```python
from build123d import *

# Parameters (mm, degrees)
BOSS_EXTRUDE1_DEPTH = 2
BOSS_EXTRUDE2_DEPTH = 22.5
SKETCH1_6_R         = 2.2
SKETCH1_6_R_2       = 1.3
BOSS_EXTRUDE3_DEPTH = 25
CUT_EXTRUDE1_DEPTH  = 25
SKETCH3_R           = 1.5
CUT_EXTRUDE2_DEPTH  = 25


with BuildPart() as part:
    # Sketch1 → Boss-Extrude1 (new body)
    with BuildSketch(Plane.XY):
        Polygon((-5, -5), (93, -5), (93, 0), (93, 56), (93, 61), (-5, 61), align=None)
    extrude(amount=BOSS_EXTRUDE1_DEPTH)

    # Sketch1_5 → Boss-Extrude2 (add)
    with BuildSketch(Plane.XY):
        with BuildLine():
            Line((-5, 63), (93, 63))
            ThreePointArc((93, 63), (94.414213562, 62.414213562), (95, 61))
            Line((95, 61), (95, 56))
            Line((95, 56), (95, 0))
            Line((95, 0), (95, -5))
            ThreePointArc((95, -5), (94.414213562, -6.414213562), (93, -7))
            Line((93, -7), (-5, -7))
            ThreePointArc((-5, -7), (-6.414213562, -6.414213562), (-7, -5))
            Line((-7, -5), (-7, 61))
            ThreePointArc((-7, 61), (-6.414213562, 62.414213562), (-5, 63))
        make_face()
        Polygon((93, 56), (93, 61), (-5, 61), (-5, -5), (93, -5), (93, 0), align=None, mode=Mode.SUBTRACT)
    extrude(amount=BOSS_EXTRUDE2_DEPTH)

    # Sketch1_6 → Boss-Extrude3 (add)
    # profile 1 of 4: a face of its own
    with BuildSketch(Plane.XY):
        with Locations((3.5, 52.5)):
            Circle(SKETCH1_6_R)
        with Locations((3.5, 52.5)):
            Circle(SKETCH1_6_R_2, mode=Mode.SUBTRACT)
    # profile 2 of 4: a face of its own
    with BuildSketch(Plane.XY):
        with Locations((61.5, 52.5)):
            Circle(SKETCH1_6_R)
        with Locations((61.5, 52.5)):
            Circle(SKETCH1_6_R_2, mode=Mode.SUBTRACT)
    # profile 3 of 4: a face of its own
    with BuildSketch(Plane.XY):
        with Locations((61.5, 3.5)):
            Circle(SKETCH1_6_R)
        with Locations((61.5, 3.5)):
            Circle(SKETCH1_6_R_2, mode=Mode.SUBTRACT)
    # profile 4 of 4: a face of its own
    with BuildSketch(Plane.XY):
        with Locations((3.5, 3.5)):
            Circle(SKETCH1_6_R)
        with Locations((3.5, 3.5)):
            Circle(SKETCH1_6_R_2, mode=Mode.SUBTRACT)
    extrude(amount=BOSS_EXTRUDE3_DEPTH)

    # Sketch2 → Cut-Extrude1 (cut)
    with BuildSketch(Plane(origin=(0, 0, 0), x_dir=(-1, 0, 0), z_dir=(0, 0, -1))):
        Polygon((-20, 20.5), (-12.5, 20.5), (-12.5, 22.5), (-18, 22.5), (-18, 28), (-18, 33.5), (-12.5, 33.5), (-12.5, 35.5), (-20, 35.5), (-27.5, 35.5), (-27.5, 33.5), (-22, 33.5), (-22, 28), (-22, 22.5), (-27.5, 22.5), (-27.5, 20.5), align=None)
    extrude(amount=-CUT_EXTRUDE1_DEPTH, mode=Mode.SUBTRACT)

    # Sketch3 → Cut-Extrude2 (cut)
    with BuildSketch(Plane.ZY.offset(7)):
        with Locations((12.31170847, 35)):
            Circle(SKETCH3_R)
        with Locations((12.31170847, 21)):
            Circle(SKETCH3_R)
    extrude(amount=-CUT_EXTRUDE2_DEPTH, mode=Mode.SUBTRACT)


solid = part.part
```
Build history of the part. All positions in model axes, mm. A direction names the side the tool comes from. Round coordinates to 2 decimals unless told otherwise and drop trailing zeros. Write each loop counter-clockwise with the first axis right and the second up, starting at its lowest first coordinate (ties: lowest second). Pieces come first, ordered by that corner, then holes.
1) Band-saw the part on D-D, the plane x = 84.5. List the corners of the cut face in (y, z), and give its area (3 significant figures).
2) Pin check, flat tips, straight feed: pin 1 (2 mm diameter, centred on x = 52.5, y = 13, fed in from +Z); pin 2 (1.8 mm diameter, centred on y = 21, z = 12.31, fed in from -X). Stop position of each tip, or through.
3) 3-axis set-ups, long thin cutter, end or side, ignore diameter. For faces 4 (the flat face through (63, 53, 25)), 5 (the flat face through (61, 4, 2)), 6 (the flat face through (12.5, 21, 1)): which of +Z, -Z, +X, -X, +Y, -Y reach the whole face in a straight line?
4) Band-saw the part on A-A, the plane z = 7.75. Give the number of separate pieces and of enclosed holes in the cut face, and give its area (3 significant figures).
5) Mould opens along Y. For faces 1 (the flat face through (3, 2, 25)), 2 (the flat face through (45, -7, 11)), 3 (the cylindrical face through (5.6, 4.16, 13.34)) say: +Y half, -Y half, draft (parallel to the pull), parting line (faces both ways), or undercut.
6) Drill centre lines: probe 1 along X at (y, z) = (3.5, 11.75); probe 2 along Y at (x, z) = (61.5, 14); probe 3 along Y at (x, z) = (68, 9). Where is each one in solid material? Low to high.
7) Band-saw the part on B-B, the plane y = 27. List the corners of the cut face in (x, z), and give its area (3 significant figures).
Ans:
1. outline: (-7, 0) - (63, 0) - (63, 22.5) - (61, 22.5) - (61, 2) - (-5, 2) - (-5, 22.5) - (-7, 22.5) - close
1. area: 222 mm2
2. pin 1: stops at z = 2
2. pin 2: stops at x = 93
3. face 4: +Z, +X, -X, +Y, -Y
3. face 5: +Z
3. face 6: +Z, -Z
4. separate pieces: 5
4. enclosed holes: 5
4. area: 708 mm2
5. face 1: draft
5. face 2: -Y half
5. face 3: undercut
6. probe 1: x = -7 to -5, 1.3 to 2.2, 4.8 to 5.7, 59.3 to 60.2, 62.8 to 63.7, 93 to 95
6. probe 2: y = -7 to -5, 1.3 to 2.2, 4.8 to 5.7, 50.3 to 51.2, 53.8 to 54.7, 61 to 63
6. probe 3: y = -7 to -5, 61 to 63
7. outline: (-7, 0) - (18, 0) - (18, 2) - (-5, 2) - (-5, 22.5) - (-7, 22.5) - close; (22, 0) - (95, 0) - (95, 22.5) - (93, 22.5) - (93, 2) - (22, 2) - close
7. area: 278 mm2
